```python
from build123d import *

# Parameters (mm, degrees)
F0_R     = 6
F0_R_2   = 4
F1_DEPTH = 2
F2_R     = 5
F2_R_2   = 4
F3_DEPTH = 2
F4_SIZE  = 0.5


with BuildPart() as f1:
    # F0 (on Top) → F1 (new body)
    with BuildSketch(Plane.XY):
        Circle(F0_R)
        Circle(F0_R_2, mode=Mode.SUBTRACT)
    extrude(amount=F1_DEPTH)

    # F2 (on face) → F3 (join)
    with BuildSketch(Plane(origin=(0, 0, 0), x_dir=(1, 0, 0), z_dir=(0, 0, -1))):
        Circle(F2_R)
        Circle(F2_R_2, mode=Mode.SUBTRACT)
    extrude(amount=F3_DEPTH)

    # F4
    f4_edges = [f1.edges().sort_by_distance(p)[0] for p in [
        (-5, 0, -2),
    ]]
    chamfer(f4_edges, length=F4_SIZE)


solid = f1.part
```
For this review, take the finished solid that the model builds, in its own axes (mm). Coordinates: 2 decimals unless noted, no trailing zeros. Write each loop counter-clockwise with the first axis right and the second up, starting at its lowest first coordinate (ties: lowest second). Pieces come first, ordered by that corner, then holes. Notation, with made-up numbers: (83, -22.5) - (124, -22.5) arc R32 ccw to (124, 7.5) - close; hole circle Ø9 at (66.25, -27). An arc over 180 degrees is marked (long way). Answer in a Markdown table with one row per item. Add a question column.
Q1. We need section C-C, the plane z = 1.55. State the section outline as (x, y) points.
Q2. We need section A-A, the plane x = 0. State the section outline as (y, z) points.
Q3. Draft analysis for pull direction Y (two halves, no side actions). For faces 1 (the flat face through (-4, 4, 0)), 2 (the cylindrical face through (-1.08, 4.88, -0.74)), 3 (the cylindrical face through (-0.867, 3.905, 0.028)), state which applies: +Y half, -Y half, draft (parallel to the pull), parting line (faces both ways), or undercut.
Q4. For P1, Ø5, axis at x = 0, y = 0, coming from the -Z side; P2, Ø2, axis at y = -3, z = 1.5, coming from the -X side, all flat-tipped, find the tip position at first contact; note any pin that passes through.
Q5. We need section D-D, the plane z = -0.7. State the section outline as (x, y) points.
Q6. For probe 1 along Y at (x, z) = (0, 0.3); probe 2 along X at (y, z) = (0, -1); probe 3 along Y at (x, z) = (1.5, 1.1), list the stretches that pass through material, from the lowest coordinate up.
Answer list:
| question | item | result |
|---|---|---|
| 1 | outline | circle Ø12 at (0, 0); hole circle Ø8 at (0, 0) |
| 2 | outline | (-6, 0) - (-5, 0) - (-5, -1.5) - (-4.5, -2) - (-4, -2) - (-4, 2) - (-6, 2) - close; (4, -2) - (4.5, -2) - (5, -1.5) - (5, 0) - (6, 0) - (6, 2) - (4, 2) - close |
| 3 | face 1 | draft |
| 3 | face 2 | parting line |
| 3 | face 3 | undercut |
| 4 | P1 | passes through |
| 4 | P2 | stops at x = -5.66 |
| 5 | outline | circle Ø10 at (0, 0); hole circle Ø8 at (0, 0) |
| 6 | probe 1 | y = -6 to -4, 4 to 6 |
| 6 | probe 2 | x = -5 to -4, 4 to 5 |
| 6 | probe 3 | y = -5.81 to -3.71, 3.71 to 5.81 |
